Autodesk Fusion 360 part; units mm, degrees
sketch "Sketch1" plane through (0, 0, 0) normal (0, 1, 0) x (1, 0, 0)
  circle A0 centre (0, 0) radius 9.7059
  line L0 (0, -9.7059) -> (0, 9.7059)
  dimension "d1" = 19.4118
revolve "Revolve1" add sketch "Sketch1" angle 360 about axis through (0, 0, 9.7059) along (0, 0, -1) contours A0 L0 picked at (2.6606, -2.8528)
sketch "Sketch2" plane through (0, 0, 0) normal (0, 1, 0) x (1, 0, 0)
  circle A0 centre (0, 0) radius 9.7059 construction
  line L0 (0, -9.7059) -> (0, 9.7059)
  line L1 (0, 9.7059) -> (5, 9.7059)
  line L2 (5, 9.7059) -> (5, 8.3189)
  line L3 (5, 8.3189) -> (2.5, 8.3189)
  line L4 (2.5, 8.3189) -> (2.5, 5.3189)
  line L5 (2.5, 5.3189) -> (0, 5.3189)
  dimension "d5" = 2.5
  dimension "d9" = 5
  dimension "d10" = 3
revolve "Revolve2" cut sketch "Sketch2" angle 360 about axis through (0, 0, 9.7059) along (0, 0, -1)
fillet "Fillet1" radius 0.4 1 edges at (-2.3308, -0.904, -8.3189)
equation "d1 = atomsize"
equation "atomsize = ( 110 / ( 170 / 30 ) ) * 1 mm"
equation "a_size = ( ( atomsize * 2 ) / ( ( 6 ) ^ ( 1 / 2 ) ) )"
Verification items for the finished model (mm, model axes). Coordinates: 2 decimals unless noted, no trailing zeros. Order: outer loops, then holes, each group sorted by start corner. A loop starts at its lowest first (then second) coordinate and runs counter-clockwise, first axis right, second up. Notation, with made-up numbers: (-34, -14.5) -> (-27, -14.5) arc R20 ccw to (-27, 14.5) -> close; hole circle Ø5 at (21, 65.5). An arc over 180 degrees is marked (long way). Use CSV: the item, a comma, the result in double quotes. Start each with the question number.
Q1. Section check D-D, the plane x = 4. Record the cut outline in (y, z), and give its area (3 significant figures).
Q2. Draft check along Y on faces 1 (the flat face through (0, 0, -5.319)), 2 (the flat face through (2.2, 2.2, -8.319)). Enter one of: +Y half, -Y half, draft (parallel to the pull), parting line (faces both ways), or undercut.
Q3. Depth check by flat-ended pin: P1, Ø1.5, axis at x = 0, y = 0.5, coming from the -Z side; P2, Ø2, axis at x = 6, y = -1.5, coming from the +Z side; P3, Ø4, axis at x = 5.5, z = -4, coming from the -Y side. Enter the tip coordinate at first touch or a pass-through.
Q4. Section check A-A, the plane z = 0. Record the cut outline in (x, y), and give its area (3 significant figures).
Q5. Thickness scan on line 1 along X through (y, z) = (0, -7.15); line 2 along X through (y, z) = (0.75, -6.5); line 3 along Y through (x, z) = (0, -6). Record the ranges inside material, lowest first.
Q6. Section check B-B, the plane x = 0. Record the cut outline in (y, z).
Returned:
1,outline,"(-3, -8.32) -> (3, -8.32) arc R8.84 ccw (long way) to start"
1,area,"244 mm^2"
2,face 1,"undercut"
2,face 2,"draft"
3,P1,"stops at z = -5.32"
3,P2,"stops at z = 8.21"
3,P3,"stops at y = -8.44"
4,outline,"circle Ø19.41 at (0, 0)"
4,area,"296 mm^2"
5,line 1,"x = -6.56 to -2.5, 2.5 to 6.56"
5,line 2,"x = -7.17 to -2.38, 2.38 to 7.17"
5,line 3,"y = -7.63 to -2.5, 2.5 to 7.63"
6,outline,"(-5, -8.32) -> (-2.9, -8.32) arc R0.4 ccw to (-2.5, -7.92) -> (-2.5, -5.32) -> (2.5, -5.32) -> (2.5, -7.92) arc R0.4 ccw to (2.9, -8.32) -> (5, -8.32) arc R9.71 ccw (long way) to start"
